Can you work these out from the model? Positions are in its coordinate system, mm. A direction names the side the tool comes from. Give positions to 0.01 mm unless a question says otherwise; leave off trailing zeros. Loops run counter-clockwise (first coordinate to the right, second up) from the corner with the lowest first, then second, coordinate; pieces in that order, holes last.
Autodesk Fusion 360 part; units mm, degrees
sketch "Sketch1" plane through (0, 0, 0) normal (0, 0, 1) x (1, 0, 0)
  line L0 (0, 0) -> (-20, 0)
  line L1 (-20, 0) -> (-20, -20)
  line L2 (-20, -20) -> (0, -20)
  line L3 (0, -20) -> (0, 0)
  line L4 (-20, 0) -> (0, 0)
  line L5 (0, 0) -> (0, 2)
  line L6 (0, 2) -> (-20, 2)
  line L7 (-20, 2) -> (-20, 0)
  dimension "d1" = 20
  dimension "d2" = 20
  dimension "d3" = 20
  dimension "d4" = 2
extrude "Extrude1" add sketch "Sketch1" along normal blind 1.8 contours L0 L1 L2 L3 L4
extrude "Extrude2" add sketch "Sketch1" along normal blind 7 contours L0 L4 L5 L6 L7
fillet "Fillet1" radius 3 2 edges at (0, 1, 7) (-20, 1, 7)
fillet "Fillet2" radius 5 2 edges at (0, -20, 0.9) (-20, -20, 0.9)
(1) Suppose I cut it at C-C on y = -11.5. List the corners of the cut face in (x, z) for me, plus the area to 3 significant figures.
Returned:
outline: (-20, 0) - (0, 0) - (0, 1.8) - (-20, 1.8) - close
area: 36.0 mm2
(2) Suppose I cut it at D-D on z = 3. List the corners of the cut face in (x, y) for me.
Returned:
outline: (-20, 0) - (0, 0) - (0, 2) - (-20, 2) - close
(3) Which directions (+Z, -Z, +X, -X, +Y, -Y) give clear straight access to the entire face, cutting with the end or side of a thin tool? Please do faces 1 (the cylindrical face through (-2, -19, 1)), 2 (the flat face through (-10, -10, 1.8)).
Returned:
face 1: +Z, -Z, +X, -Y
face 2: +Z, +X, -X, -Y
(4) Please list where these lines run through material, in increasing order: probe 1 along Y at (x, z) = (-10.75, 3); probe 2 along Z at (x, y) = (-19, -1.5); probe 3 along Y at (x, z) = (-2, 1).
Returned:
probe 1: y = 0 to 2
probe 2: z = 0 to 1.8
probe 3: y = -19 to 2
(5) Suppose I cut it at B-B on z = 1. List the corners of the cut face in (x, y) for me.
Returned:
outline: (-20, -15) arc R5 ccw to (-15, -20) - (-5, -20) arc R5 ccw to (0, -15) - (0, 2) - (-20, 2) - close
(6) Suppose I cut it at A-A on x = -9. List the corners of the cut face in (y, z) for me.
Returned:
outline: (-20, 0) - (2, 0) - (2, 7) - (0, 7) - (0, 1.8) - (-20, 1.8) - close
(7) Will these pins go through, and if not, where does the flat tip stop? P1, Ø2.5, axis at x = -5.5, z = 5.5, coming from the -Y side; P2, Ø8, axis at x = -8.5, y = -17, coming from the +Z side.
Returned:
P1: stops at y = 0
P2: stops at z = 1.8
